The listing builds one solid part. Answer for the finished solid, in the listing's coordinates (mm). A direction names the side the tool comes from. Give positions to 0.01 mm unless a question says otherwise; leave off trailing zeros. Loops run counter-clockwise (first coordinate to the right, second up) from the corner with the lowest first, then second, coordinate; pieces in that order, holes last. Notation, with made-up numbers: M -19.5,86.5 L -5.5,86.5 A20 ccw -5.5,111.5 Z; hole C 68,15 d8. An arc over 180 degrees is marked long. Return JSON: item names as keys, results as strings.
from build123d import *

# Parameters (mm, degrees)
SKETCH1_R               = 45
BOSS_EXTRUDE1_DEPTH     = 2.5
SKETCH2_R               = 45
SKETCH2_R_2             = 42.5
BOSS_EXTRUDE2_DEPTH     = 4.5
SKETCH3_R               = 8
CUT_EXTRUDE1_DEPTH      = 10
SKETCH5_R               = 13.5
SKETCH5_R_2             = 11
BOSS_EXTRUDE3_DEPTH     = 5
SKETCH7_W               = 43.18
SKETCH7_H               = 17.78
CUT_EXTRUDE2_DEPTH      = 0.5
CUT_EXTRUDE3_DEPTH      = 5
CUT_EXTRUDE4_DEPTH      = 0.5
SKETCH11_R              = 13.5
SKETCH11_R_2            = 8
BOSS_EXTRUDE4_DEPTH     = 2.8
SKETCH14_R              = 2.625
CUT_EXTRUDE5_DEPTH      = 6
CUT_EXTRUDE5_DEPTH_BACK = 3.5
FILLET1_R               = 2.5


with BuildPart() as part:
    # Sketch1 → Boss-Extrude1 (new body)
    with BuildSketch(Plane.XY):
        Circle(SKETCH1_R)
    extrude(amount=BOSS_EXTRUDE1_DEPTH)

    # Sketch2 → Boss-Extrude2 (add)
    with BuildSketch(Plane.XY.offset(2.5)):
        Circle(SKETCH2_R)
        Circle(SKETCH2_R_2, mode=Mode.SUBTRACT)
    extrude(amount=BOSS_EXTRUDE2_DEPTH)

    # Sketch3 → Cut-Extrude1 (cut)
    with BuildSketch(Plane.XY.offset(2.5)):
        Circle(SKETCH3_R)
    extrude(amount=-CUT_EXTRUDE1_DEPTH, mode=Mode.SUBTRACT)

    # Sketch5 → Boss-Extrude3 (add)
    with BuildSketch(Plane.XY.offset(2.5)):
        Circle(SKETCH5_R)
        Circle(SKETCH5_R_2, mode=Mode.SUBTRACT)
    extrude(amount=BOSS_EXTRUDE3_DEPTH)

    # Sketch7 → Cut-Extrude2 (cut)
    with BuildSketch(Plane.XY.offset(2.5)):
        with Locations((0, 26)):
            Rectangle(SKETCH7_W, SKETCH7_H)
    extrude(amount=-CUT_EXTRUDE2_DEPTH, mode=Mode.SUBTRACT)

    # Sketch8 → Cut-Extrude3 (cut)
    with BuildSketch(Plane.XY.offset(2.5)):
        Polygon((-16.496556405, -12.72805329), (-11.002519002, -24.510054522), (-25.503443595, -31.27194671), (-30.997480998, -19.489945478), align=None)
    extrude(amount=-CUT_EXTRUDE3_DEPTH, mode=Mode.SUBTRACT)

    # Sketch9 → Cut-Extrude4 (cut)
    with BuildSketch(Plane(origin=(0, 0, 0), x_dir=(-1, 0, 0), z_dir=(0, 0, -1))):
        Polygon((27.250107322, -13.32900476), (27.884034715, -11.969543079), (29.923227236, -12.920434168), (30.874118325, -10.881241647), (32.233580005, -11.51516904), (31.282688916, -13.554361561), (33.321881437, -14.505252649), (32.687954045, -15.86471433), (30.648761524, -14.913823241), (29.697870435, -16.953015762), (28.338408754, -16.319088369), (29.289299843, -14.279895849), align=None)
        Polygon((18.187029452, -9.102822142), (18.820956845, -7.743360462), (24.258803567, -10.279070032), (23.624876174, -11.638531713), align=None)
    extrude(amount=-CUT_EXTRUDE4_DEPTH, mode=Mode.SUBTRACT)

    # Sketch11 → Boss-Extrude4 (add)
    with BuildSketch(Plane.XY.offset(2.5)):
        Circle(SKETCH11_R)
        Circle(SKETCH11_R_2, mode=Mode.SUBTRACT)
    extrude(amount=BOSS_EXTRUDE4_DEPTH)

    # Sketch14 → Cut-Extrude5 (cut, two sides)
    with BuildSketch(Plane.XY.offset(2.5)) as cut_extrude5_sk:
        with Locations((0, -32.5)):
            Circle(SKETCH14_R)
        with Locations((-28.145825623, 16.25)):
            Circle(SKETCH14_R)
        with Locations((28.145825623, 16.25)):
            Circle(SKETCH14_R)
    extrude(amount=CUT_EXTRUDE5_DEPTH, mode=Mode.SUBTRACT)
    extrude(cut_extrude5_sk.sketch, amount=-CUT_EXTRUDE5_DEPTH_BACK, mode=Mode.SUBTRACT)

    # Fillet1
    fillet1_edges = [part.edges().sort_by_distance(p)[0] for p in [
        (-13.5, 0, 2.5),
    ]]
    fillet(fillet1_edges, radius=FILLET1_R)


solid = part.part
(1) Determine the mould class of faces 1 (the cylindrical face through (20.765, -39.923, 3.451)), 2 (the flat face through (-26.9, -33.1, 7)), 3 (the flat face through (-1, -18, 2.5)) for opening direction Y: released by +Y, released by -Y, zero draft, split by the parting line, or undercut.
Values follow:
{"face 1": "split by the parting line", "face 2": "zero draft", "face 3": "undercut"}
(2) The part is cut by section C-C (x = -20). Determine the outline of the cut face in (y, z), and give its area (3 significant figures).
Values follow:
{"outline": "M -40.31,0 L -28.71,0 L -28.71,2.5 L -37.5,2.5 L -37.5,7 L -40.31,7 Z; M -14.36,0 L -9.95,0 L -9.95,0.5 L -8.29,0.5 L -8.29,0 L 40.31,0 L 40.31,7 L 37.5,7 L 37.5,2.5 L 34.89,2.5 L 34.89,2 L 17.11,2 L 17.11,2.5 L -14.36,2.5 Z", "area": "181 mm²"}
(3) The part is cut by section D-D (y = 37). Determine the outline of the cut face in (x, z), and give its area (3 significant figures).
Values follow:
{"outline": "M -25.61,0 L 25.61,0 L 25.61,7 L 20.91,7 L 20.91,2.5 L -20.91,2.5 L -20.91,7 L -25.61,7 Z", "area": "170 mm²"}
(4) The part is cut by section B-B (x = 0). Give the number of separate pieces and of enclosed holes in the cut face, and give its area (3 significant figures).
Values follow:
{"separate pieces": "3", "enclosed holes": "0", "area": "230 mm²"}
(5) The part is cut by section A-A (y = 0). Determine the outline of the cut face in (x, z).
Values follow:
{"outline": "M -45,0 L -8,0 L -8,5.3 L -11,5.3 L -11,7.5 L -13.5,7.5 L -13.5,5 A2.5 cw -16,2.5 L -42.5,2.5 L -42.5,7 L -45,7 Z; M 8,0 L 45,0 L 45,7 L 42.5,7 L 42.5,2.5 L 16,2.5 A2.5 cw 13.5,5 L 13.5,7.5 L 11,7.5 L 11,5.3 L 8,5.3 Z"}
(6) A tool of negligible diameter and unlimited length cuts with its end or side. For faces 4 (the flat face through (-5, -10, 7.5)), 5 (the flat face through (-21, -10, 0.5)), 6 (the flat face through (-18.151, -27.844, 1.268)), 7 (the cylindrical face through (-2.38, -10.74, 6.38)), 8 (the flat face through (9, 1, 0)), from which of +Z, -Z, +X, -X, +Y, -Y can it reach the whole face along a straight path? Write none if from no direction.
Values follow:
{"face 4": "+Z, +X, -X, +Y, -Y", "face 5": "-Z", "face 6": "+Z, -Z", "face 7": "+Z", "face 8": "-Z, +X, -X, +Y, -Y"}
(7) Given pin 1 (1.5 mm diameter, centred on x = 31, z = 1, fed in from +Y); pin 2 (2 mm diameter, centred on y = 3.5, z = 3.5, fed in from +X); pin 3 (6.5 mm diameter, centred on x = 0, y = 5, fed in from +Z), each flat-ended and moving along its own axis, determine where each tip first touches the part or whether it passes through.
Values follow:
{"pin 1": "y = 33.32", "pin 2": "x = 44.93", "pin 3": "z = 5.3"}
(8) Straight lines are drawn through the part: line 1 along Y through (x, z) = (0, 5.45); line 2 along X through (y, z) = (-6, 3.5); line 3 along Z through (x, y) = (24.5, 28). For each, find the intervals that lie inside material, in ascending order.
Values follow:
{"line 1": "-45 to -42.5, -13.5 to -11, 11 to 13.5, 42.5 to 45", "line 2": "-44.6 to -42.07, -12.65 to -5.29, 5.29 to 12.65, 42.07 to 44.6", "line 3": "0 to 2.5"}
